Build history of the part. All positions in model axes, mm. A direction names the side the tool comes from. Give positions to 0.01 mm unless a question says otherwise; leave off trailing zeros. Order: outer loops, then holes, each group sorted by start corner. A loop starts at its lowest first (then second) coordinate and runs counter-clockwise, first axis right, second up. Notation, with made-up numbers: M 50.5,85 L 85.5,85 A16 cw 85.5,109 Z; hole C 72,-21 d5. An arc over 180 degrees is marked long. Use CSV: the item, a comma, the result in double quotes. Start each with the question number.
Item 1: Pin check, flat tips, straight feed: P1, Ø4.5, axis at x = -22.5, z = 6.5, coming from the -Y side; P2, Ø3, axis at x = 30, y = 1.5, coming from the -Z side; P3, Ø12, axis at x = -0.5, z = 10, coming from the +Y side; P4, Ø5, axis at y = 10, z = 14.5, coming from the +X side. Stop position of each tip, or through.
Item 2: Band-saw the part on B-B on x = -10. Write the cut outline in (y, z).
Item 3: Band-saw the part on C-C on x = -22. Write the cut outline in (y, z), plus the area to 3 significant figures.
Item 4: Band-saw the part on A-A on y = -2.5. Write the cut outline in (x, z), plus the area to 3 significant figures.
Item 5: Two-plate mould, pull along Y, no slides. Class faces 1 (the flat face through (2, -29, 10)), 2 (the flat face through (-2, 9, 1)), 3 (the flat face through (12, 8, 10)): pulls with the +Y half, pulls with the -Y half, needs draft (parallel to the pull), parting line crosses it, or undercut.
Item 6: Wall check: line 1 along X through (y, z) = (11.8, 10); line 2 along X through (y, z) = (9.5, 10); line 3 along Y through (x, z) = (21, 12.25). Give the ranges that are in metal, low to high.
Item 7: Which spindle directions (+Z, -Z, +X, -X, +Y, -Y) get a long thin tool onto all of the face, cutting with end or side? Do faces 4 (the flat face through (-17.725, -14, 10)), 5 (the flat face through (-12.725, 9, 2)), 6 (the flat face through (-25, 2, 5.971)), 7 (the cylindrical face through (22.01, 9.48, 10.27)). Say none if no direction does.
from build123d import *

# Parameters (mm, degrees)
SKETCH1_W            = 57
SKETCH1_H            = 20
BOSS_EXTRUDE2_DEPTH  = 3
SKETCH3_W            = 40
SKETCH3_H            = 20
BOSS_EXTRUDE3_DEPTH  = 27
SKETCH4_W            = 40
SKETCH4_H            = 20
BOSS_EXTRUDE4_DEPTH  = 5
SKETCH7_R            = 2.049783944
BOSS_EXTRUDE5_DEPTH  = 3
SKETCH8_W            = 40
SKETCH8_H            = 20
BOSS_EXTRUDE6_DEPTH  = 2
FILLET1_R            = 2
FILLET3_R            = 1
CUT_EXTRUDE1_DEPTH   = 12
CUT_EXTRUDE2_DEPTH   = 12
SKETCH12_R           = 2.049783944
BOSS_EXTRUDE7_DEPTH  = 10
SKETCH13_W           = 38
SKETCH13_H           = 0.1
CUT_EXTRUDE3_DEPTH   = 0.1
SKETCH14_W           = 18
SKETCH14_H           = 0.1
CUT_EXTRUDE4_DEPTH   = 0.1
SKETCH16_W           = 18
SKETCH16_H           = 0.1
BOSS_EXTRUDE10_DEPTH = 0.1
BOSS_EXTRUDE13_DEPTH = 0.5
SKETCH18_R           = 5.505741297
SKETCH18_R_2         = 4.954025226
BOSS_EXTRUDE14_DEPTH = 0.5
BOSS_EXTRUDE15_DEPTH = 0.5
SKETCH22_R           = 2.049783944
BOSS_EXTRUDE17_DEPTH = 0.01


with BuildPart() as part:
    # Sketch1 → Boss-Extrude2 (new body)
    with BuildSketch(Plane(origin=(0, 0, 0), x_dir=(1, 0, 0), z_dir=(0, 1, 0))):
        with Locations((2.775361092, -10)):
            Rectangle(SKETCH1_W, SKETCH1_H)
    extrude(amount=BOSS_EXTRUDE2_DEPTH)

    # Sketch3 → Boss-Extrude3 (add)
    with BuildSketch(Plane.XZ):
        with Locations((2.275361092, 10)):
            Rectangle(SKETCH3_W, SKETCH3_H)
    extrude(amount=BOSS_EXTRUDE3_DEPTH)

    # Sketch4 → Boss-Extrude4 (add)
    with BuildSketch(Plane(origin=(0, 3, 0), x_dir=(1, 0, 0), z_dir=(0, 1, 0))):
        with Locations((2.275361092, -10)):
            Rectangle(SKETCH4_W, SKETCH4_H)
    extrude(amount=BOSS_EXTRUDE4_DEPTH)

    # Sketch7 → Boss-Extrude5 (add)
    with BuildSketch(Plane(origin=(0, 8, 0), x_dir=(1, 0, 0), z_dir=(0, 1, 0))):
        with BuildLine():
            Line((8.555331619, -1), (-12.724638908, -1))
            Line((-12.724638908, -1), (-12.724638908, -4))
            ThreePointArc((-12.724638908, -4), (-15.83010298, -10), (-12.724638908, -16))
            Line((-12.724638908, -16), (-12.724638908, -19))
            Line((-12.724638908, -19), (8.555331619, -19))
            ThreePointArc((8.555331619, -19), (22.013873261, -10), (8.555331619, -1))
        make_face()
        with Locations(Location((12.275361092, -10, 0), (0, 0, 270))):
            Circle(SKETCH7_R, mode=Mode.SUBTRACT)
    extrude(amount=BOSS_EXTRUDE5_DEPTH)

    # Sketch8 → Boss-Extrude6 (add)
    with BuildSketch(Plane.XZ.offset(27)):
        with Locations((2.275361092, 10)):
            Rectangle(SKETCH8_W, SKETCH8_H)
    extrude(amount=BOSS_EXTRUDE6_DEPTH)

    # Fillet1
    fillet1_edges = [part.edges().sort_by_distance(p)[0] for p in [
        (2.275361092, -29, 20),
        (2.275361092, -29, 0),
    ]]
    fillet(fillet1_edges, radius=FILLET1_R)

    # Fillet3
    fillet3_edges = [part.edges().sort_by_distance(p)[0] for p in [
        (22.275361092, -29, 10),
        (-17.724638908, -29, 10),
        (-17.724638908, -13.5, 0),
        (-17.724638908, -13.5, 20),
        (-17.724638908, -28.414213562, 0.585786438),
        (-17.724638908, -28.414213562, 19.414213562),
        (22.275361092, -13.5, 20),
        (22.275361092, -13.5, 0),
        (22.275361092, -28.414213562, 0.585786438),
        (22.275361092, -28.414213562, 19.414213562),
    ]]
    fillet(fillet3_edges, radius=FILLET3_R)

    # Sketch9 → Cut-Extrude1 (cut)
    with BuildSketch(Plane(origin=(0, 3, 0), x_dir=(1, 0, 0), z_dir=(0, 1, 0))):
        with BuildLine():
            Line((-25.724638908, -15.974539408), (-25.724638908, -14.029117413))
            Line((-25.724638908, -14.029117413), (-23.473177442, -14.029117413))
            ThreePointArc((-23.473177442, -14.029117413), (-19.724640003, -14.997907425), (-23.47114197, -15.974539408))
            Line((-23.47114197, -15.974539408), (-25.724638908, -15.974539408))
        make_face()
        with BuildLine():
            Line((-23.47114197, -4.025460592), (-25.724638908, -4.025460592))
            Line((-25.724638908, -4.025460592), (-25.724638908, -5.970882587))
            Line((-25.724638908, -5.970882587), (-23.473177442, -5.970882587))
            ThreePointArc((-23.473177442, -5.970882587), (-19.724640003, -5.002092575), (-23.47114197, -4.025460592))
        make_face()
    extrude(amount=-CUT_EXTRUDE1_DEPTH, mode=Mode.SUBTRACT)

    # Sketch11 → Cut-Extrude2 (cut)
    with BuildSketch(Plane(origin=(0, 3, 0), x_dir=(1, 0, 0), z_dir=(0, 1, 0))):
        with BuildLine():
            Line((31.275361092, -5.46228452), (31.275361092, -4.46228452))
            Line((31.275361092, -4.46228452), (28.711852765, -4.46228452))
            ThreePointArc((28.711852765, -4.46228452), (24.775361092, -4.96228452), (28.711852765, -5.46228452))
            Line((28.711852765, -5.46228452), (31.275361092, -5.46228452))
        make_face()
        with BuildLine():
            Line((28.711852765, -14.53771548), (31.275361092, -14.53771548))
            Line((31.275361092, -14.53771548), (31.275361092, -15.53771548))
            Line((31.275361092, -15.53771548), (28.711852765, -15.53771548))
            ThreePointArc((28.711852765, -15.53771548), (24.775361092, -15.03771548), (28.711852765, -14.53771548))
        make_face()
    extrude(amount=-CUT_EXTRUDE2_DEPTH, mode=Mode.SUBTRACT)

    # Sketch13 → Cut-Extrude3 (cut)
    with BuildSketch(Plane.XY.offset(20)):
        with Locations((2.275361092, -0.05)):
            Rectangle(SKETCH13_W, SKETCH13_H)
    extrude(amount=-CUT_EXTRUDE3_DEPTH, mode=Mode.SUBTRACT)

    # Sketch14 → Cut-Extrude4 (cut)
    with BuildSketch(Plane(origin=(22.275361092, 0, 0), x_dir=(0, 0, -1), z_dir=(1, 0, 0))):
        with Locations((-10, -0.05)):
            Rectangle(SKETCH14_W, SKETCH14_H)
    extrude(amount=-CUT_EXTRUDE4_DEPTH, mode=Mode.SUBTRACT)

    # Sketch16 → Boss-Extrude10 (add)
    with BuildSketch(Plane.ZY.offset(17.724638908)):
        with Locations((10, -0.05)):
            Rectangle(SKETCH16_W, SKETCH16_H)
    extrude(amount=BOSS_EXTRUDE10_DEPTH)



with BuildPart() as body_2:
    # Sketch12 → Boss-Extrude7 (new body)
    with BuildSketch(Plane(origin=(0, 11, 0), x_dir=(1, 0, 0), z_dir=(0, 1, 0))):
        with Locations(Location((12.275361092, -10, 0), (0, 0, 270))):
            Circle(SKETCH12_R)
    extrude(amount=BOSS_EXTRUDE7_DEPTH)


with BuildPart() as part_1:
    add(part.part)

    add(body_2.part)  # Boss-Extrude13 merges body 2
    # Sketch17 → Boss-Extrude13 (add)
    with BuildSketch(Plane(origin=(0, 11, 0), x_dir=(1, 0, 0), z_dir=(0, 1, 0))):
        with BuildLine():
            Line((20.850118946, -10.288863052), (19.089941192, -10.454244634))
            ThreePointArc((19.089941192, -10.454244634), (18.190057204, -13.414851392), (16.076038534, -15.674477166))
            Line((16.076038534, -15.674477166), (16.81290276, -17.281526608))
            ThreePointArc((16.81290276, -17.281526608), (16.707171545, -17.676120875), (16.312577278, -17.57038966))
            Line((16.312577278, -17.57038966), (15.289263749, -16.1287218))
            ThreePointArc((15.289263749, -16.1287218), (12.275361092, -16.829702785), (9.261458434, -16.1287218))
            Line((9.261458434, -16.1287218), (8.238144905, -17.57038966))
            ThreePointArc((8.238144905, -17.57038966), (7.843550638, -17.676120875), (7.737819423, -17.281526608))
            Line((7.737819423, -17.281526608), (8.474683649, -15.674477166))
            ThreePointArc((8.474683649, -15.674477166), (6.360664979, -13.414851392), (5.460780991, -10.454244634))
            Line((5.460780991, -10.454244634), (3.700603237, -10.288863052))
            ThreePointArc((3.700603237, -10.288863052), (3.411740185, -10), (3.700603237, -9.711136948))
            Line((3.700603237, -9.711136948), (5.460780991, -9.545755366))
            ThreePointArc((5.460780991, -9.545755366), (6.360664979, -6.585148608), (8.474683649, -4.325522834))
            Line((8.474683649, -4.325522834), (7.737819423, -2.718473392))
            ThreePointArc((7.737819423, -2.718473392), (7.843550638, -2.323879125), (8.238144905, -2.42961034))
            Line((8.238144905, -2.42961034), (9.261458434, -3.8712782))
            ThreePointArc((9.261458434, -3.8712782), (12.275361092, -3.170297215), (15.289263749, -3.8712782))
            Line((15.289263749, -3.8712782), (16.312577278, -2.42961034))
            ThreePointArc((16.312577278, -2.42961034), (16.707171545, -2.323879125), (16.81290276, -2.718473392))
            Line((16.81290276, -2.718473392), (16.076038534, -4.325522834))
            ThreePointArc((16.076038534, -4.325522834), (18.190057204, -6.585148608), (19.089941192, -9.545755366))
            Line((19.089941192, -9.545755366), (20.850118946, -9.711136948))
            ThreePointArc((20.850118946, -9.711136948), (21.138981999, -10), (20.850118946, -10.288863052))
        make_face()
    extrude(amount=BOSS_EXTRUDE13_DEPTH)

    # Sketch18 → Boss-Extrude14 (add)
    with BuildSketch(Plane(origin=(0, 11.5, 0), x_dir=(1, 0, 0), z_dir=(0, 1, 0))):
        with Locations(Location((12.275361092, -10, 0), (0, 0, 270))):
            Circle(SKETCH18_R)
        with Locations(Location((12.275361092, -10, 0), (0, 0, 270))):
            Circle(SKETCH18_R_2, mode=Mode.SUBTRACT)
    extrude(amount=BOSS_EXTRUDE14_DEPTH)

    # Sketch20 → Boss-Extrude15 (add)
    with BuildSketch(Plane(origin=(0, 11, 0), x_dir=(1, 0, 0), z_dir=(0, 1, 0))):
        with BuildLine():
            Line((-1.482591904, -18), (-1.482591904, -2))
            Line((-1.482591904, -2), (-11.724638908, -2))
            Line((-11.724638908, -2), (-11.724638908, -4.542063407))
            ThreePointArc((-11.724638908, -4.542063407), (-14.83010298, -10), (-11.724638908, -15.457936593))
            Line((-11.724638908, -15.457936593), (-11.724638908, -18))
            Line((-11.724638908, -18), (-1.482591904, -18))
        make_face()
        with BuildLine():
            Line((-2.482591904, -3), (-10.724638908, -3))
            Line((-10.724638908, -3), (-10.724638908, -5.144266923))
            ThreePointArc((-10.724638908, -5.144266923), (-13.83010298, -10), (-10.724638908, -14.855733077))
            Line((-10.724638908, -14.855733077), (-10.724638908, -17))
            Line((-10.724638908, -17), (-2.482591904, -17))
            Line((-2.482591904, -17), (-2.482591904, -3))
        make_face(mode=Mode.SUBTRACT)
    extrude(amount=BOSS_EXTRUDE15_DEPTH)

    # Sketch22 → Boss-Extrude17 (add)
    with BuildSketch(Plane(origin=(0, 21, 0), x_dir=(1, 0, 0), z_dir=(0, 1, 0))):
        with Locations(Location((12.275361092, -10, 0), (0, 0, 270))):
            Circle(SKETCH22_R)
    extrude(amount=BOSS_EXTRUDE17_DEPTH)


solid = part_1.part
Model answer:
1,P1,"stops at y = 0"
1,P2,"stops at z = 0"
1,P3,"stops at y = 11.5"
1,P4,"stops at x = 22.28"
2,outline,"M -29,2 A2 ccw -27,0 L 8,0 L 8,1 L 11,1 L 11,2 L 11.5,2 L 11.5,3 L 11,3 L 11,17 L 11.5,17 L 11.5,18 L 11,18 L 11,19 L 8,19 L 8,20 L 0,20 L 0,19.9 L -0.1,19.9 L -0.1,20 L -27,20 A2 ccw -29,18 Z"
3,outline,"M 0,0 L 3,0 L 3,3.02 L 0,3.02 Z; M 0,6.98 L 3,6.98 L 3,13.02 L 0,13.02 Z; M 0,16.98 L 3,16.98 L 3,20 L 0,20 Z"
3,area,"36.2 mm^2"
4,outline,"M -17.72,1 A1 ccw -16.72,0 L 21.28,0 A1 ccw 22.28,1 L 22.28,19 A1 ccw 21.28,20 L -16.72,20 A1 ccw -17.72,19 Z"
4,area,"799 mm^2"
5,face 1,"pulls with the -Y half"
5,face 2,"needs draft"
5,face 3,"undercut"
6,line 1,"x = 6.77 to 7.32, 10.23 to 14.33, 17.23 to 17.78"
6,line 2,"x = -15.83 to 10.23, 14.33 to 22.01"
6,line 3,"y = -29 to 11"
7,face 4,"+Z, -Z, -X, -Y"
7,face 5,"-Z, -X, +Y"
7,face 6,"-X, +Y, -Y"
7,face 7,"+Y"
